The listing builds one solid part. Answer for the finished solid, in the listing's coordinates (mm). Face numbers are marked on the shaded views. A direction names the side the tool comes from. Give positions to 0.01 mm unless a question says otherwise; leave off trailing zeros. Write each loop counter-clockwise with the first axis right and the second up, starting at its lowest first coordinate (ties: lowest second). Pieces come first, ordered by that corner, then holes. Notation, with made-up numbers: (-2.75, -24) - (12.25, -24) arc R21 cw to (12.25, 7) - close; hole circle Ø4 at (-13, 22). An arc over 180 degrees is marked (long way). Answer in a Markdown table with one row per item. Add a question column.
from build123d import *

# Parameters (mm, degrees)
F1_DEPTH = 63.5
F2_DEPTH = 7.9375
F0_W     = 25.3758770108
F0_H     = 19.05
F3_DEPTH = 25.4
F5_R     = 6.35


with BuildPart() as f1:
    # F0 (on Front) → F1 (new body, symmetric)
    with BuildSketch(Plane.XZ):
        Polygon((-41.275, 9.525), (-41.275, -9.525), (41.275, -9.525), (41.275, 9.525), (22.225, 9.525), align=None)
    extrude(amount=F1_DEPTH, both=True)

    # F0 (on Front) → F2 (join, symmetric)
    with BuildSketch(Plane.XZ):
        with BuildLine():
            add(Edge.make_bspline(
                [(-41.275, 9.525), (-41.3212813437, 39.7789143026), (21.7138361186, 62.3522996902), (57.15, 61.9252)],
                knots=[0, 0, 0, 0, 111.5045361635, 111.5045361635, 111.5045361635, 111.5045361635], degree=3))
            Line((-41.275, 9.525), (22.225, 9.525))
            Line((22.225, 9.525), (22.225, 27.0002))
            ThreePointArc((22.225, 27.0002), (32.4542956671, 51.6959043329), (57.15, 61.9252))
        make_face()
    extrude(amount=F2_DEPTH, both=True)

    # F0 (on Front) → F3 (join, symmetric)
    with BuildSketch(Plane.XZ):
        with Locations((73.0129385054, 52.4002)):
            Rectangle(F0_W, F0_H)
        with BuildLine():
            Line((22.225, 9.525), (41.275, 9.525))
            Line((41.275, 9.525), (41.275, 27.0002))
            ThreePointArc((41.275, 27.0002), (45.9246798487, 38.2255201513), (57.15, 42.8752))
            Line((57.15, 42.8752), (60.325, 42.8752))
            Line((60.325, 42.8752), (60.325, 61.9252))
            Line((60.325, 61.9252), (57.15, 61.9252))
            ThreePointArc((57.15, 61.9252), (32.4542956671, 51.6959043329), (22.225, 27.0002))
            Line((22.225, 27.0002), (22.225, 9.525))
        make_face()
    extrude(amount=F3_DEPTH, both=True)

    # F0 (on Front) → F4 (revolve)
    with BuildSketch(Plane.XZ):
        Polygon((85.7008770108, 66.675), (85.7008770108, 61.9252), (85.7008770108, 42.8752), (85.7008770108, 38.1), (111.125, 38.1), (111.125, 66.675), align=None)
    revolve(axis=Axis((85.7008770108, 0, 52.3875), (0, 0, -1)))

    # F5
    f5_edges = [f1.edges().sort_by_distance(p)[0] for p in [
        (41.275, -63.5, 0),
        (-41.275, -63.5, 0),
        (41.275, 63.5, 0),
        (-41.275, 63.5, 0),
    ]]
    fillet(f5_edges, radius=F5_R)


solid = f1.part
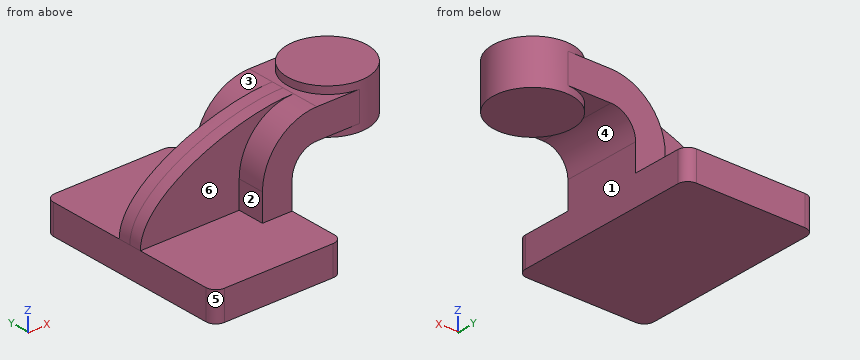
1. Section A-A (z = -1.5) is taken. Give the vertices of the cut face in (x, y) (3 decimals), and give its area (3 significant figures).
2. Straight lines are drawn through the part: L1, parallel to X at y = -24.5, z = 1 (3 decimals); L2, parallel to Z at x = -14, y = -14.5 (3 decimals); L3, parallel to Y at x = 30, z = 30.5. For each, find the intervals that lie inside material, in ascending order. Write a range as [from, to].
3. A tool of negligible diameter and unlimited length cuts with its end or side. For the marked faces 1, 2 and 3, from which of +Z, -Z, +X, -X, +Y, -Y can it reach the whole face along a straight path? Write none if from no direction.
4. Section B-B (y = 28) is taken. Give the vertices of the cut face in (x, z) (3 decimals), and give its area (3 significant figures).
5. Given pin 1 Ø15.5 at (x, z) = (47.5, 47) entering from -Y; pin 2 Ø2 at (x, y) = (66.5, -21.5) entering from +Z; pin 3 Ø2 at (x, z) = (-1.5, 35.5) entering from -Y, each flat-ended and moving along its own axis, determine where each tip first touches the part or whether it passes through.
6. Section C-C (x = 101.5) is taken. Give the vertices of the cut face in (y, z) (3 decimals), and give its area (3 significant figures).
7. The mould has two halves that part along X. Classify the marked faces 4, 5 and 6: +X half, -X half, draft (parallel to the pull), parting line (faces both ways), or undercut.
Geometry check:
| question | item | result |
|---|---|---|
| 1 | outline | (-41.275, -57.15) arc R6.35 ccw to (-34.925, -63.5) - (34.925, -63.5) arc R6.35 ccw to (41.275, -57.15) - (41.275, 57.15) arc R6.35 ccw to (34.925, 63.5) - (-34.925, 63.5) arc R6.35 ccw to (-41.275, 57.15) - close |
| 1 | area | 10,400 mm² |
| 2 | L1 | [-41.275, 41.275] |
| 2 | L2 | [-9.525, 9.525] |
| 2 | L3 | [-25.4, 25.4] |
| 3 | face 1 | -Z, +X, +Y, -Y |
| 3 | face 2 | +Z, -X, -Y |
| 3 | face 3 | +Z, -X, +Y |
| 4 | outline | (-41.275, -9.525) - (41.275, -9.525) - (41.275, 9.525) - (-41.275, 9.525) - close |
| 4 | area | 1,570 mm² |
| 5 | pin 1 | y = -25.4 |
| 5 | pin 2 | z = 61.93 |
| 5 | pin 3 | y = -7.94 |
| 6 | outline | (-19.919, 38.1) - (19.919, 38.1) - (19.919, 66.675) - (-19.919, 66.675) - close |
| 6 | area | 1,140 mm² |
| 7 | face 4 | undercut |
| 7 | face 5 | -X half |
| 7 | face 6 | draft |
